Here's how the part is built. I have some questions about the finished solid (model axes, mm). Face numbers are marked on the shaded views. Coordinates: 2 decimals unless noted, no trailing zeros. Write each loop counter-clockwise with the first axis right and the second up, starting at its lowest first coordinate (ties: lowest second). Pieces come first, ordered by that corner, then holes.
Item 1: I want a section at B-B (z = -60). Please give me the cut outline in (x, y), and give its area (3 significant figures).
Item 2: I want a section at C-C (z = -15). Please give me the cut outline in (x, y), and give its area (3 significant figures).
Item 3: I want a section at A-A (x = 26). Please give me the cut outline in (y, z).
Item 4: I'm going to push flat-ended pins straight in: P1, Ø4, axis at x = 58.5, z = -51, coming from the +Y side; P2, Ø3, axis at x = 86.5, z = 85, coming from the +Y side. Where does each tip first touch, or does it pass through?
Item 5: If we mould it in two halves opening along Z, with no side actions, what happens to the marked faces 1 and 2? For each: pulls with the +Z half, pulls with the -Z half, needs draft (parallel to the pull), parting line crosses it, or undercut.
Item 6: Please list where these lines run through material, in increasing order: line 1 (X direction, y = 12, z = -85); line 2 (X direction, y = 6, z = -85); line 3 (X direction, y = -0.25, z = -1).
from build123d import *

# Parameters (mm, degrees)
SKETCH_1_W          = 200
SKETCH_1_H          = 200
SKETCH_1_R          = 5
EXTRUDE_1_DEPTH     = 7
SKETCH_2_R          = 10
SKETCH_2_R_2        = 5
EXTRUDE_2_DEPTH     = 15
SKETCH_3_W          = 200
SKETCH_3_H          = 200
EXTRUDE_3_DEPTH     = 3
CUT_EXTRUDE_2_DEPTH = 143.214626533
FILLET_2_R          = 5


with BuildPart() as part:
    # 草圖1 → 填料-伸長1 (new body)
    with BuildSketch(Plane(origin=(0, 0, 0), x_dir=(1, 0, 0), z_dir=(0, 1, 0))):
        Rectangle(SKETCH_1_W, SKETCH_1_H)
        with Locations(Location((85, 85, 0), (0, 0, 270))):
            Circle(SKETCH_1_R, mode=Mode.SUBTRACT)
        with Locations(Location((-85, 85, 0), (0, 0, 90))):
            Circle(SKETCH_1_R, mode=Mode.SUBTRACT)
        with Locations(Location((85, -85, 0), (0, 0, 90))):
            Circle(SKETCH_1_R, mode=Mode.SUBTRACT)
        with Locations(Location((-85, -85, 0), (0, 0, 270))):
            Circle(SKETCH_1_R, mode=Mode.SUBTRACT)
    extrude(amount=EXTRUDE_1_DEPTH)

    # 草圖2 → 填料-伸長2 (add)
    # profile 1 of 4: a face of its own
    with BuildSketch(Plane(origin=(0, 7, 0), x_dir=(1, 0, 0), z_dir=(0, 1, 0))):
        with Locations(Location((-85, 85, 0), (0, 0, 90))):
            Circle(SKETCH_2_R)
        with Locations(Location((-85, 85, 0), (0, 0, 90))):
            Circle(SKETCH_2_R_2, mode=Mode.SUBTRACT)
    # profile 2 of 4: a face of its own
    with BuildSketch(Plane(origin=(0, 7, 0), x_dir=(1, 0, 0), z_dir=(0, 1, 0))):
        with Locations(Location((85, 85, 0), (0, 0, 90))):
            Circle(SKETCH_2_R)
        with Locations(Location((85, 85, 0), (0, 0, 270))):
            Circle(SKETCH_2_R_2, mode=Mode.SUBTRACT)
    # profile 3 of 4: a face of its own
    with BuildSketch(Plane(origin=(0, 7, 0), x_dir=(1, 0, 0), z_dir=(0, 1, 0))):
        with Locations(Location((85, -85, 0), (0, 0, 90))):
            Circle(SKETCH_2_R)
        with Locations(Location((85, -85, 0), (0, 0, 90))):
            Circle(SKETCH_2_R_2, mode=Mode.SUBTRACT)
    # profile 4 of 4: a face of its own
    with BuildSketch(Plane(origin=(0, 7, 0), x_dir=(1, 0, 0), z_dir=(0, 1, 0))):
        with Locations(Location((-85, -85, 0), (0, 0, 90))):
            Circle(SKETCH_2_R)
        with Locations(Location((-85, -85, 0), (0, 0, 270))):
            Circle(SKETCH_2_R_2, mode=Mode.SUBTRACT)
    extrude(amount=EXTRUDE_2_DEPTH)

    # 草圖3 → 填料-伸長3 (add)
    with BuildSketch(Plane.XZ):
        Rectangle(SKETCH_3_W, SKETCH_3_H)
    extrude(amount=EXTRUDE_3_DEPTH)

    # 草圖6 → 除料-伸長2 (cut, through all)
    with BuildSketch(Plane(origin=(0, 7, 0), x_dir=(1, 0, 0), z_dir=(0, 1, 0))):
        Polygon((-67.5, 85.991963893), (0, 25.991963893), (67.5, 85.991963893), align=None)
        Polygon((85.991963893, -67.5), (85.991963893, 67.5), (35.991963893, 0), align=None)
        Polygon((-67.5, -85.991963893), (67.5, -85.991963893), (0, -25.991963893), align=None)
        Polygon((-85.991963893, 67.5), (-85.991963893, -67.5), (-35.991963893, 0), align=None)
    extrude(amount=-CUT_EXTRUDE_2_DEPTH, mode=Mode.SUBTRACT)

    # 圓角2
    fillet_2_edges = [part.edges().sort_by_distance(p)[0] for p in [
        (-67.5, 2, -85.991963893),
        (67.5, 2, -85.991963893),
        (0, 2, -25.991963893),
        (-85, 7, -75),
        (85, 7, -75),
        (85, 7, 95),
        (-85, 7, 95),
        (0, 2, 25.991963893),
        (67.5, 2, 85.991963893),
        (-67.5, 2, 85.991963893),
        (35.991963893, 2, 0),
        (85.991963893, 2, -67.5),
        (85.991963893, 2, 67.5),
        (-35.991963893, 2, 0),
        (-85.991963893, 2, 67.5),
        (-85.991963893, 2, -67.5),
    ]]
    fillet(fillet_2_edges, radius=FILLET_2_R - 0.0001)  # a hair under: the kernel refuses the full size


solid = part.part
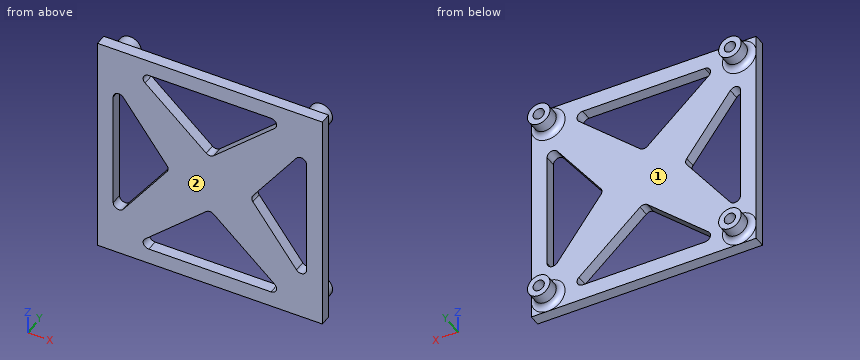
Answer:
1. outline: (-100, -3) - (-38.26, -3) - (-38.26, 7) - (-100, 7) - close; (38.26, -3) - (100, -3) - (100, 7) - (38.26, 7) - close
1. area: 1,230 mm2
2. outline: (-100, -3) - (-85.99, -3) - (-85.99, 7) - (-100, 7) - close; (-47.1, -3) - (47.1, -3) - (47.1, 7) - (-47.1, 7) - close; (85.99, -3) - (100, -3) - (100, 7) - (85.99, 7) - close
2. area: 1,220 mm2
3. outline: (-3, -100) - (7, -100) - (7, -85.99) - (-3, -85.99) - close; (-3, -49.1) - (7, -49.1) - (7, 49.1) - (-3, 49.1) - close; (-3, 85.99) - (7, 85.99) - (7, 100) - (-3, 100) - close
4. P1: stops at y = 7
4. P2: stops at y = 0
5. face 1: undercut
5. face 2: needs draft
6. line 1: x = -95 to -90, -80 to -75, 75 to 80, 90 to 95
6. line 2: x = -100 to -90, -80 to -57.34, 57.34 to 80, 90 to 100
6. line 3: x = -100 to -85.99, -37.32 to 37.32, 85.99 to 100
